Autodesk Inventor part; units mm, degrees
ref_plane "YZ Plane" through (0, 0, 0) normal (1, 0, 0) x (0, 1, 0)
ref_plane "XZ Plane" through (0, 0, 0) normal (0, 1, 0) x (-1, 0, 0)
ref_plane "XY Plane" through (0, 0, 0) normal (0, 0, 1) x (1, 0, 0)
sketch "Sketch1" plane through (0, 0, 0) normal (1, 0, 0) x (0, 1, 0)
  line L0 (12.7, 0) -> (38.1, 0)
  line L1 (50.8, -12.7) -> (50.8, -139.7)
  line L2 (38.1, -152.4) -> (12.7, -152.4)
  line L3 (0, -139.7) -> (0, -12.7)
  arc A0 (50.8, -12.7) -> (38.1, 0) centre (38.1, -12.7) ccw
  arc A1 (12.7, 0) -> (0, -12.7) centre (12.7, -12.7) ccw
  arc A2 (0, -139.7) -> (12.7, -152.4) centre (12.7, -139.7) ccw
  arc A3 (38.1, -152.4) -> (50.8, -139.7) centre (38.1, -139.7) ccw
  circle A4 centre (25.4, -28.575) radius 14.2875
  circle A5 centre (25.4, -60.325) radius 6.35
  circle A6 centre (25.4, -92.075) radius 6.35
  circle A7 centre (25.4, -123.825) radius 6.35
  circle A8 centre (25.4, -123.825) radius 22 construction
  circle A9 centre (40.9563, -139.3813) radius 1.75
  circle A10 centre (40.9563, -108.2687) radius 1.75
  circle A11 centre (9.8437, -108.2687) radius 1.75
  circle A12 centre (9.8437, -139.3813) radius 1.75
  line L4 (25.4, -28.575) -> (25.4, -123.825) construction
  point P0 (0, 0)
  point P1 (50.8, -152.4)
  point P2 (50.8, 0)
  point P3 (0, -152.4)
  point P4 (25.4, -152.4)
  point P5 (25.4, -76.2)
  point P6 (0, -76.2)
  dimension "d10" = 44
  dimension "d0" = 50.8
  dimension "d1" = 152.4
  dimension "d2" = 12.7
  dimension "d3" = 28.575
  dimension "d4" = 12.7
  dimension "d5" = 12.7
  dimension "d6" = 12.7
  dimension "d7" = 31.75
  dimension "d8" = 31.75
  dimension "d9" = 31.75
  dimension "d11" = 3.5
  dimension "d14" = 360
extrude "Extrusion1" add sketch "Sketch1" along normal blind 3.175
equation "\"d8\" = d7"
equation "\"d9\" = d7"
properties part number "Housing"
For this review, take the finished solid that the model builds, in its own axes (mm). Round coordinates to 2 decimals unless told otherwise and drop trailing zeros. Write each loop counter-clockwise with the first axis right and the second up, starting at its lowest first coordinate (ties: lowest second). Pieces come first, ordered by that corner, then holes.
1) For line 1 along Z through (x, y) = (1.6, 25.4) (1 decimal); line 2 along Z through (x, y) = (0.35, 24); line 3 along Y through (x, z) = (2.6, -22), list the stretches that pass through material, from the lowest coordinate up.
Answer below:
line 1: z = -152.4 to -130.2, -117.5 to -98.4, -85.7 to -66.7, -54 to -42.9, -14.3 to 0
line 2: z = -152.4 to -130.02, -117.63 to -98.27, -85.88 to -66.52, -54.13 to -42.79, -14.36 to 0
line 3: y = 0 to 12.72, 38.08 to 50.8
2) Insertion check: pin 1 Ø14.5 at (y, z) = (25.4, -92.075) entering from -X; pin 2 Ø3 at (y, z) = (9.84, -108.27) entering from -X. Each pin has a flat end and moves straight along its axis. Give the tip position at first contact, or say it passes through.
Answer below:
pin 1: stops at x = 0
pin 2: passes through
3) Take a section at C-C on x = 1. State how many separate pieces and enclosed holes the cut face has, then the cut area to 3 significant figures.
Answer below:
separate pieces: 1
enclosed holes: 8
area: 6,540 mm2
4) Take a section at B-B on z = -90.5. Give the boundary of the cut face in (x, y) (3 decimals).
Answer below:
outline: (0, 0) - (3.175, 0) - (3.175, 19.248) - (0, 19.248) - close; (0, 31.552) - (3.175, 31.552) - (3.175, 50.8) - (0, 50.8) - close
5) Mouldability with a two-part tool opening along Y and no side actions: class faces 1 (the face through (1.565, 24.023, -85.876)), 2 (the face through (2, 50.8, -75)), 3 (the face through (2, 0, -77)) as +Y half, -Y half, draft (parallel to the pull), parting line (faces both ways), or undercut.
Answer below:
face 1: undercut
face 2: +Y half
face 3: -Y half
6) Take a section at A-A on y = 25.4. Give the boundary of the cut face in (x, z) (1 decimal), then the cut area to 3 significant figures.
Answer below:
outline: (0, -152.4) - (3.2, -152.4) - (3.2, -130.2) - (0, -130.2) - close; (0, -117.5) - (3.2, -117.5) - (3.2, -98.4) - (0, -98.4) - close; (0, -85.7) - (3.2, -85.7) - (3.2, -66.7) - (0, -66.7) - close; (0, -54) - (3.2, -54) - (3.2, -42.9) - (0, -42.9) - close; (0, -14.3) - (3.2, -14.3) - (3.2, 0) - (0, 0) - close
area: 272 mm2
